```python
from build123d import *

# Parameters (mm, degrees)
SKETCH1_R               = 30
BOSS_EXTRUDE1_DEPTH     = 6
SKETCH2_R               = 14.5
BOSS_EXTRUDE2_DEPTH     = 13
CUT_EXTRUDE1_DEPTH      = 47.486557197
CUT_EXTRUDE1_DEPTH_BACK = 47.486557197
SKETCH3_R               = 12.75
BOSS_EXTRUDE4_START     = 13
SKETCH5_R               = 30
SKETCH5_R_2             = 12.75
BOSS_EXTRUDE4_DEPTH     = 6
CUT_EXTRUDE2_DEPTH      = 45.373415465
CUT_EXTRUDE2_DEPTH_BACK = 45.373415465
SKETCH6_R               = 2
CUT_EXTRUDE3_DEPTH      = 47.486557197
CUT_EXTRUDE3_DEPTH_BACK = 47.486557197
FILLET1_R               = 2
FILLET2_R               = 2
FILLET3_R               = 2
FILLET4_R               = 2
SKETCH8_R               = 4
BOSS_EXTRUDE5_DEPTH     = 13
FILLET5_R               = 2
FILLET6_R               = 2
FILLET7_R               = 2
FILLET8_R               = 2


with BuildPart() as part:
    # Sketch1 → Boss-Extrude1 (new body)
    with BuildSketch(Plane.XY):
        Circle(SKETCH1_R)
    extrude(amount=-BOSS_EXTRUDE1_DEPTH)

    # Sketch2 → Boss-Extrude2 (add)
    with BuildSketch(Plane.XY):
        with Locations(Location((0, 0, 0), (0, 0, 180))):
            Circle(SKETCH2_R)
    extrude(amount=BOSS_EXTRUDE2_DEPTH)

    # Sketch3 → Cut-Extrude1 (cut, two sides: drawn at the far end of the back side and taken through both)
    with BuildSketch(Plane.XY.offset(13).offset(-CUT_EXTRUDE1_DEPTH_BACK)):
        Circle(SKETCH3_R)
    extrude(amount=CUT_EXTRUDE1_DEPTH + CUT_EXTRUDE1_DEPTH_BACK, mode=Mode.SUBTRACT)

    # Sketch5 → Boss-Extrude4 (add)
    with BuildSketch(Plane.XY.offset(BOSS_EXTRUDE4_START)):
        Circle(SKETCH5_R)
        Circle(SKETCH5_R_2, mode=Mode.SUBTRACT)
    extrude(amount=-BOSS_EXTRUDE4_DEPTH)

    # Sketch6 → Cut-Extrude2 (cut, two sides: drawn at the far end of the back side and taken through both)
    with BuildSketch(Plane.XY.offset(-CUT_EXTRUDE2_DEPTH_BACK)):
        with Locations((-20.333162568, -12.75)):
            Circle(SKETCH6_R)
        with Locations((-22.659159296, 12.75)):
            Circle(SKETCH6_R)
        with Locations((20.333162568, -12.75)):
            Circle(SKETCH6_R)
        with Locations((22.659159296, 12.75)):
            Circle(SKETCH6_R)
    extrude(amount=CUT_EXTRUDE2_DEPTH + CUT_EXTRUDE2_DEPTH_BACK, mode=Mode.SUBTRACT)

    # Sketch7 → Cut-Extrude3 (cut, two sides: drawn at the far end of the back side and taken through both)
    with BuildSketch(Plane.XY.offset(13).offset(-CUT_EXTRUDE3_DEPTH_BACK)):
        with BuildLine():
            Line((10.445298657, -12.448222201), (19.283628291, -22.981333294))
            ThreePointArc((19.283628291, -22.981333294), (0, -30), (-19.283628291, -22.981333294))
            Line((-19.283628291, -22.981333294), (-10.445298657, -12.448222201))
            ThreePointArc((-10.445298657, -12.448222201), (0, -16.25), (10.445298657, -12.448222201))
        make_face()
        with BuildLine():
            Line((-10.445298657, 12.448222201), (-19.283628291, 22.981333294))
            ThreePointArc((-19.283628291, 22.981333294), (0, 30), (19.283628291, 22.981333294))
            Line((19.283628291, 22.981333294), (10.445298657, 12.448222201))
            ThreePointArc((10.445298657, 12.448222201), (0, 16.25), (-10.445298657, 12.448222201))
        make_face()
    extrude(amount=CUT_EXTRUDE3_DEPTH + CUT_EXTRUDE3_DEPTH_BACK, mode=Mode.SUBTRACT)

    # Fillet1
    fillet1_edges = [part.edges().sort_by_distance(p)[0] for p in [
        (-19.283628291, -22.981333294, 10),
    ]]
    fillet(fillet1_edges, radius=FILLET1_R)

    # Fillet2
    fillet2_edges = [part.edges().sort_by_distance(p)[0] for p in [
        (-19.283628291, 22.981333294, 10),
    ]]
    fillet(fillet2_edges, radius=FILLET2_R)

    # Fillet3
    fillet3_edges = [part.edges().sort_by_distance(p)[0] for p in [
        (19.283628291, 22.981333294, 10),
    ]]
    fillet(fillet3_edges, radius=FILLET3_R)

    # Fillet4
    fillet4_edges = [part.edges().sort_by_distance(p)[0] for p in [
        (19.283628291, -22.981333294, 10),
    ]]
    fillet(fillet4_edges, radius=FILLET4_R)

    # Sketch8 → Boss-Extrude5 (add)
    with BuildSketch(Plane.XY.offset(13)):
        with Locations((-22, 0)):
            Circle(SKETCH8_R)
        with Locations((22, 0)):
            Circle(SKETCH8_R)
    extrude(amount=-BOSS_EXTRUDE5_DEPTH)

    # Fillet5
    fillet5_edges = [part.edges().sort_by_distance(p)[0] for p in [
        (-19.283628291, 22.981333294, -3),
    ]]
    fillet(fillet5_edges, radius=FILLET5_R)

    # Fillet6
    fillet6_edges = [part.edges().sort_by_distance(p)[0] for p in [
        (-19.283628291, -22.981333294, -3),
    ]]
    fillet(fillet6_edges, radius=FILLET6_R)

    # Fillet7
    fillet7_edges = [part.edges().sort_by_distance(p)[0] for p in [
        (19.283628291, -22.981333294, -3),
    ]]
    fillet(fillet7_edges, radius=FILLET7_R)

    # Fillet8
    fillet8_edges = [part.edges().sort_by_distance(p)[0] for p in [
        (19.283628291, 22.981333294, -3),
    ]]
    fillet(fillet8_edges, radius=FILLET8_R)


solid = part.part
```
Verification items for the finished model (mm, model axes). A direction names the side the tool comes from. Coordinates: 2 decimals unless noted, no trailing zeros. Order: outer loops, then holes, each group sorted by start corner. A loop starts at its lowest first (then second) coordinate and runs counter-clockwise, first axis right, second up. Notation, with made-up numbers: (11, -7) - (44, -7) arc R11 cw to (44, 5) - close; hole circle Ø11 at (84.5, 25.25). An arc over 180 degrees is marked (long way). Return JSON: item names as keys, results as strings.
(1) Section check C-C, the plane z = 11.25. Record the cut outline in (x, y), and give its area (3 significant figures).
Filled sheet:
{"outline": "(-20.88, -21.55) arc R2 ccw to (-17.95, -21.39) - (-10.45, -12.45) arc R16.25 ccw to (10.45, -12.45) - (17.95, -21.39) arc R2 ccw to (20.88, -21.55) arc R30 ccw to (20.88, 21.55) arc R2 ccw to (17.95, 21.39) - (10.45, 12.45) arc R16.25 ccw to (-10.45, 12.45) - (-17.95, 21.39) arc R2 ccw to (-20.88, 21.55) arc R30 ccw to start; hole circle Ø4 at (-22.66, 12.75); hole circle Ø4 at (-20.33, -12.75); hole circle Ø25.5 at (0, 0); hole circle Ø4 at (20.33, -12.75); hole circle Ø4 at (22.66, 12.75)", "area": "1,370 mm^2"}
(2) Thickness scan on line 1 along Z through (x, y) = (22, -14.5); line 2 along Y through (x, z) = (0, 4); line 3 along X through (y, z) = (0.5, -1.75). Record the ranges inside material, lowest first.
Filled sheet:
{"line 1": "z = -6 to 0, 7 to 13", "line 2": "y = -14.5 to -12.75, 12.75 to 14.5", "line 3": "x = -30 to -12.74, 12.74 to 30"}
(3) Section check B-B, the plane x = 0. Record the cut outline in (y, z).
Filled sheet:
{"outline": "(-16.25, -6) - (-12.75, -6) - (-12.75, 13) - (-16.25, 13) - (-16.25, 7) - (-14.5, 7) - (-14.5, 0) - (-16.25, 0) - close; (12.75, -6) - (16.25, -6) - (16.25, 0) - (14.5, 0) - (14.5, 7) - (16.25, 7) - (16.25, 13) - (12.75, 13) - close"}
(4) Go/stop test with flat-tipped pins: pin 1 (4 mm diameter, centred on y = -3, z = 1.5, fed in from +X); pin 2 (5 mm diameter, centred on y = -13, z = 8, fed in from -X); pin 3 (3 mm diameter, centred on x = 22.66, y = 12.75, fed in from -Z); pin 4 (4 mm diameter, centred on x = 0, z = -2.5, fed in from +Y). Record where each tip stops, or that it passes through.
Filled sheet:
{"pin 1": "stops at x = 29.95", "pin 2": "stops at x = -28.1", "pin 3": "passes through", "pin 4": "stops at y = 16.25"}
(5) Section check D-D, the plane y = 18.5. Record the cut outline in (x, z), and give its area (3 significant figures).
Filled sheet:
{"outline": "(-23.62, -6) - (-15.52, -6) - (-15.52, 0) - (-23.62, 0) - close; (-23.62, 7) - (-15.52, 7) - (-15.52, 13) - (-23.62, 13) - close; (15.52, -6) - (23.62, -6) - (23.62, 0) - (15.52, 0) - close; (15.52, 7) - (23.62, 7) - (23.62, 13) - (15.52, 13) - close", "area": "194 mm^2"}
(6) Mould release check, pull along Z, two halves, no side actions. Record for faces 1 (the cylindrical face through (-6.691, 12.864, 3.451)), 2 (the flat face through (13, 0, -6)), 3 (the cylindrical face through (-2.764, -12.447, 3.367)): pulls with the +Z half, pulls with the -Z half, needs draft (parallel to the pull), parting line crosses it, or undercut.
Filled sheet:
{"face 1": "undercut", "face 2": "pulls with the -Z half", "face 3": "needs draft"}
(7) Section check A-A, the plane y = 0. Record the cut outline in (x, z).
Filled sheet:
{"outline": "(-30, -6) - (-12.75, -6) - (-12.75, 13) - (-30, 13) - (-30, 7) - (-26, 7) - (-26, 0) - (-30, 0) - close; (12.75, -6) - (30, -6) - (30, 0) - (26, 0) - (26, 7) - (30, 7) - (30, 13) - (12.75, 13) - close; hole (-18, 0) - (-14.5, 0) - (-14.5, 7) - (-18, 7) - close; hole (14.5, 0) - (18, 0) - (18, 7) - (14.5, 7) - close"}
(8) Access from +Z, -Z, +X, -X, +Y, -Y to the whole of each face (thin tool, end or side, straight path). Record for faces 4 (the flat face through (-14.146, 16.859, 9.958)), 5 (the flat face through (14.146, -16.859, -3.042)), 6 (the cylindrical face through (30, 0, 10)), 7 (the cylindrical face through (-25.2, -2.4, 3.5)), 8 (the cylindrical face through (24.567, 13.351, -3.042)).
Filled sheet:
{"face 4": "+Z, -Z, +Y", "face 5": "+Z, -Z, -Y", "face 6": "+Z, -Z, +X", "face 7": "none", "face 8": "+Z, -Z"}
